from build123d import *

# Parameters (mm, degrees)
F0_R     = 76.2
F0_R_2   = 6.35
F0_R_3   = 12.7
F1_DEPTH = 6.35


with BuildPart() as f1:
    # F0 (on Front) → F1 (new body)
    with BuildSketch(Plane.XZ):
        Circle(F0_R)
        with Locations((-35.921024, -35.921024)):
            Circle(F0_R_2, mode=Mode.SUBTRACT)
        with Locations((35.921024, -35.921024)):
            Circle(F0_R_2, mode=Mode.SUBTRACT)
        with Locations((-35.921024, 35.921024)):
            Circle(F0_R_2, mode=Mode.SUBTRACT)
        Circle(F0_R_3, mode=Mode.SUBTRACT)
        with Locations((35.921024, 35.921024)):
            Circle(F0_R_2, mode=Mode.SUBTRACT)
    extrude(amount=F1_DEPTH)


solid = f1.part
Model file for the job. Use its own axes, mm. Coordinates: 2 decimals unless noted, no trailing zeros. Order: outer loops, then holes, each group sorted by start corner. A loop starts at its lowest first (then second) coordinate and runs counter-clockwise, first axis right, second up. Notation, with made-up numbers: (86, 31) -> (137, 31) arc R21 cw to (137, 52) -> close; hole circle Ø1 at (76.25, 74). An arc over 180 degrees is marked (long way). Return JSON: item names as keys, results as strings. Group by question number.
Item 1: Flat gauge pins, fed straight in: P1, Ø2, axis at y = -3.5, z = 46, coming from the -X side; P2, Ø3, axis at x = 8.5, y = -1, coming from the +Z side; P3, Ø1, axis at y = -1, z = 46, coming from the -X side; P4, Ø7.5, axis at x = -35.92, z = -35.92, coming from the +Y side. Where does each tip first touch, or does it go through?
Item 2: Saw through at C-C on x = -34. Write the cut outline in (y, z), then the cut area to 3 significant figures.
Item 3: Saw through at A-A on z = 0. Write the cut outline in (x, y), then the cut area to 3 significant figures.
Item 4: Wall check: line 1 along Z through (x, y) = (0, -1.75); line 2 along Z through (x, y) = (-32.5, -1.5); line 3 along X through (y, z) = (-5.25, 33). Give the ranges that are in metal, low to high. Write a range as [from, to].
Item 5: Saw through at B-B on x = 0. Write the cut outline in (y, z).
Item 6: Pull direction Z, two halves, no side cores. Call faces 1 (the cylindrical face through (-2.75, -3.13, -12.4)), 2 (the cylindrical face through (-60.47, -3.131, -46.367)), 3 (the flat face through (16, 0, 1)), 4 (the cylindrical face through (-32.507, -3.131, -30.567)): pulls with the +Z half, pulls with the -Z half, needs draft (parallel to the pull), parting line crosses it, or undercut.
Item 7: Saw through at D-D on y = -5.25. Write the cut outline in (x, z), then the cut area to 3 significant figures.
Values found:
{
 "1": {"P1": "stops at x = -61.49", "P2": "stops at z = 75.88", "P3": "stops at x = -61.12", "P4": "passes through"},
 "2": {"outline": "(-6.35, -68.19) -> (0, -68.19) -> (0, -41.97) -> (-6.35, -41.97) -> close; (-6.35, -29.87) -> (0, -29.87) -> (0, 29.87) -> (-6.35, 29.87) -> close; (-6.35, 41.97) -> (0, 41.97) -> (0, 68.19) -> (-6.35, 68.19) -> close", "area": "712 mm2"},
 "3": {"outline": "(-76.2, -6.35) -> (-12.7, -6.35) -> (-12.7, 0) -> (-76.2, 0) -> close; (12.7, -6.35) -> (76.2, -6.35) -> (76.2, 0) -> (12.7, 0) -> close", "area": "806 mm2"},
 "4": {"line 1": "z = [-76.2, -12.7], [12.7, 76.2]", "line 2": "z = [-68.92, -41.27], [-30.57, 30.57], [41.27, 68.92]", "line 3": "x = [-68.68, -41.56], [-30.28, 30.28], [41.56, 68.68]"},
 "5": {"outline": "(-6.35, -76.2) -> (0, -76.2) -> (0, -12.7) -> (-6.35, -12.7) -> close; (-6.35, 12.7) -> (0, 12.7) -> (0, 76.2) -> (-6.35, 76.2) -> close"},
 "6": {"face 1": "undercut", "face 2": "parting line crosses it", "face 3": "needs draft", "face 4": "undercut"},
 "7": {"outline": "circle Ø152.4 at (0, 0); hole circle Ø12.7 at (-35.92, -35.92); hole circle Ø12.7 at (-35.92, 35.92); hole circle Ø25.4 at (0, 0); hole circle Ø12.7 at (35.92, -35.92); hole circle Ø12.7 at (35.92, 35.92)", "area": "17,200 mm2"}
}
